Can you work these out from the model? Positions are in its coordinate system, mm. A direction names the side the tool comes from. Give positions to 0.01 mm unless a question says otherwise; leave off trailing zeros. Write each loop counter-clockwise with the first axis right and the second up, starting at its lowest first coordinate (ties: lowest second). Pieces come first, ordered by that corner, then holes.
from build123d import *

# Parameters (mm, degrees)
F0_R     = 14.478
F1_DEPTH = 14.9225
F2_R     = 1.27


with BuildPart() as f1:
    # F0 (on Top) → F1 (new body)
    with BuildSketch(Plane.XY):
        Polygon((10.077578, 13.870596), (0, 25.4), (-10.077578, 13.870596), (-24.156836, 7.849032), (-16.305864, -5.298096), (-14.929745, -20.549032), (0, -17.145), (14.929745, -20.549032), (16.305864, -5.298096), (24.156836, 7.849032), align=None)
        Circle(F0_R, mode=Mode.SUBTRACT)
    extrude(amount=F1_DEPTH)

    # F2
    f2_edges = [f1.edges().sort_by_distance(p)[0] for p in [
        (-14.929745, -20.549032, 7.46125),
        (14.929745, -20.549032, 7.46125),
        (-24.156836, 7.849032, 7.46125),
        (24.156836, 7.849032, 7.46125),
        (0, 25.4, 7.46125),
        (-16.305864, -5.298096, 7.46125),
        (0, -17.145, 7.46125),
        (16.305864, -5.298096, 7.46125),
        (10.077578, 13.870596, 7.46125),
        (-10.077578, 13.870596, 7.46125),
    ]]
    fillet(f2_edges, radius=F2_R)


solid = f1.part
(1) For faces 1 (the face through (-19.982, 0.858, 7.357)), 2 (the face through (-6.99, -18.74, 7.36)), which set-ups out of +Z, -Z, +X, -X, +Y, -Y let a thin tool reach every point of the face, with its end or its side?
Returned:
face 1: +Z, -Z, -X, -Y
face 2: +Z, -Z, -Y
(2) If I drill on L1, parallel to Y at x = 0, z = 6.25; L2, parallel to Y at x = -6, z = 14.25; L3, parallel to X at y = 3.5, z = 11.75, over which ranges is the centre line in solid material (lowest first)?
Returned:
L1: y = -17.18 to -14.48, 14.48 to 24.74
L2: y = -18.51 to -13.18, 13.18 to 18.54
L3: x = -21.56 to -14.05, 14.05 to 21.56
(3) Will these pins go through, and if not, where does the flat tip stop? P1, Ø1.5, axis at y = -13, z = 9, coming from the -X side; P2, Ø8, axis at y = 2, z = 6, coming from the +X side.
Returned:
P1: stops at x = -15.68
P2: stops at x = 23.05
(4) Imagine slicing it at B-B, the plane y = 0. Write out the boundary of the cut face in (x, z).
Returned:
outline: (-19.47, 0) - (-14.48, 0) - (-14.48, 14.92) - (-19.47, 14.92) - close; (14.48, 0) - (19.47, 0) - (19.47, 14.92) - (14.48, 14.92) - close
(5) Imagine slicing it at C-C, the plane z = 9. Write out the boundary of the cut face in (x, y), plus the area to 3 significant figures.
Returned:
outline: (-23.41, 6.6) - (-16.45, -5.05) arc R1.27 cw to (-16.28, -5.59) - (-15.06, -19.1) arc R1.27 ccw to (-13.51, -20.23) - (-0.28, -17.21) arc R1.27 cw to (0.28, -17.21) - (13.51, -20.23) arc R1.27 ccw to (15.06, -19.1) - (16.28, -5.59) arc R1.27 cw to (16.45, -5.05) - (23.41, 6.6) arc R1.27 ccw to (22.82, 8.42) - (10.34, 13.76) arc R1.27 cw to (9.89, 14.09) - (0.96, 24.31) arc R1.27 ccw to (-0.96, 24.31) - (-9.89, 14.09) arc R1.27 cw to (-10.34, 13.76) - (-22.82, 8.42) arc R1.27 ccw to start; hole circle Ø28.96 at (0, 0)
area: 619 mm2
(6) If we mould it in two halves opening along X, with no side actions, what happens to faces 3 (the face through (-23.525, 7.66, 7.566)), 4 (the face through (-1.885, 14.355, 7.357)), 5 (the face through (19.88, 0.69, 7.36)), 6 (the face through (-14.1, 4, 14.922))? For each: +X half, -X half, draft (parallel to the pull), parting line (faces both ways), or undercut.
Returned:
face 3: -X half
face 4: undercut
face 5: +X half
face 6: draft
(7) Imagine slicing it at A-A, the plane x = 7. Write out the boundary of the cut face in (y, z), plus the area to 3 significant figures.
Returned:
outline: (-18.74, 0) - (-12.67, 0) - (-12.67, 14.92) - (-18.74, 14.92) - close; (12.67, 0) - (17.39, 0) - (17.39, 14.92) - (12.67, 14.92) - close
area: 161 mm2
(8) Imagine slicing it at D-D, the plane y = 16. Write out the boundary of the cut face in (x, z).
Returned:
outline: (-8.22, 0) - (8.22, 0) - (8.22, 14.92) - (-8.22, 14.92) - close
